Source: CAD feature listing. Evaluate the final solid. Frame: model axes, mm. A direction names the side the tool comes from. Give positions to 0.01 mm unless a question says otherwise; leave off trailing zeros. Write each loop counter-clockwise with the first axis right and the second up, starting at its lowest first coordinate (ties: lowest second). Pieces come first, ordered by that corner, then holes. Notation, with made-up numbers: (88, -40) -> (101, -40) arc R8 ccw to (101, -26) -> close; hole circle Ø1 at (-10, -7.5). An arc over 180 degrees is marked (long way). Write item = value, one per line.
Autodesk Inventor part; units mm, degrees
ref_plane "YZ Plane" through (0, 0, 0) normal (1, 0, 0) x (0, 1, 0)
ref_plane "XY Plane" through (0, 0, 0) normal (0, 0, 1) x (1, 0, 0)
ref_plane "UCS1: YZ Plane" through (0, 0, 0) normal (1, 0, 0) x (0, 1, 0)
sketch "Sketch2" plane through (0, 0, 0) normal (1, 0, 0) x (0, 1, 0)
  circle A0 centre (0, -70) radius 26
  line L0 (25, -200) -> (-25, -200)
  line L1 (0, -70) -> (0, -200) construction
  line L2 (-25.9992, -70.2001) -> (-25, -200)
  line L3 (25.9992, -70.2001) -> (25, -200)
  circle A1 centre (0, 0) radius 17.5
  circle A2 centre (0, -70) radius 17.5
  line L4 (17.5, 0) -> (17.5, -70)
  line L5 (-17.5, 0) -> (-17.5, -70)
  dimension "d1" = 52
  dimension "d3" = 50
  dimension "d25" = 130
  dimension "d26" = 35
  dimension "d27" = 70
extrude "Extrusion1" add sketch "Sketch2" against normal blind 45 contours A0 L5 A2 L4 | A0 L4 A2 L5 | A2
extrude "Extrusion2" add sketch "Sketch2" along normal blind 45 from surface at -45 contours A0 L3 L0 L2
sketch "Sketch5" plane through (-45, -25, -200) normal (0, 0, -1) x (-1, 0, 0)
  circle A0 centre (-22.5, 25) radius 10
  line L0 (-45, 50) -> (-45, 0)
  line L1 (-45, 50) -> (0, 50)
  point P0 (-45, 25)
  point P1 (-45, 25)
  point P2 (45, 0)
  point P3 (-22.5, 50)
  dimension "d22" = 20
extrude "Extrusion4" cut sketch "Sketch5" against normal blind 60
ref_plane "Work Plane1" through (-22.5, 0, -70) normal (1, 0, 0) x (0, 0, -1)
sketch "Sketch4" plane through (-22.5, 0, -70) normal (1, 0, 0) x (0, 0, -1)
  line L0 (130, 25) -> (130, -25)
  arc A0 (125.9592, -40) -> (130, 0) centre (-70, 0) ccw
  line L1 (125.9592, -40) -> (130, -40)
  line L2 (130, -40) -> (130, 0)
  line L3 (201.2, 0) -> (-115.2, 0)
  line L4 (-70, 0) -> (130, 0)
  point P0 (-70, 0)
  point P1 (156, -25)
  point P2 (156, 25)
  point P3 (156, -25)
  point P4 (-25, -130)
  point P5 (25, -130)
  dimension "d18" = 40
revolve "Revolution1" cut sketch "Sketch4" angle 360 about axis through (-22.5, 0, 0) along (0, 0, -1)
extrude "Extrusion5" add sketch "Sketch2" along normal blind 12 contours L5 A1 L4 A0 | A0 L4 A2 L5 | A1 | A2 picked at (-13.2429, -51.1519)
properties part number "shank_inventor"
(1) Access query for faces 5 (the face through (6, 17.5, -35)), 6 (the face through (5.916, 0.385, -87.496)), 7 (the face through (12, 0, -34)), 8 (the face through (6, -17.5, -35)). Directions: +Z, -Z, +X, -X, +Y, -Y. A direction counts if a zero-diameter tool reaches every point of the face in a straight line with its end or side. Return the directions, or none.
Values follow:
face_5 = +Z, -Z, +X, +Y
face_6 = -Z, +X
face_7 = +Z, -Z, +X, +Y, -Y
face_8 = +Z, -Z, +X, -Y
(2) Section query A-A (z = -32). Return loops of the section in (x, y).
Values follow:
outline = (0, -17.5) -> (12, -17.5) -> (12, 17.5) -> (0, 17.5) -> close
(3) Pull-direction query (Y, two-part tool) for faces 1 (the face through (5.916, -0.385, 17.496)), 2 (the face through (-22, 0, -140)), 3 (the face through (-32.04, 3, -170.29)), 4 (the face through (0, 0, -16)); classes: pulls with the +Y half, pulls with the -Y half, needs draft (parallel to the pull), parting line crosses it, or undercut.
Values follow:
face_1 = parting line crosses it
face_2 = undercut
face_3 = undercut
face_4 = needs draft
(4) Material intervals for line 1 (X direction, y = 0, z = -156); line 2 (X direction, y = 23.5, z = -184.5); line 3 (X direction, y = -12, z = -17.5), sorted ascending.
Values follow:
line_1 = -45 to -32.5, -12.5 to 0
line_2 = -45 to 0
line_3 = 0 to 12
(5) First-contact query: pin 1 (6 mm diameter, centred on x = -26, z = -169, fed in from +Y); pin 2 (9.5 mm diameter, centred on x = 4.5, z = -35.5, fed in from +Y); pin 3 (1.5 mm diameter, centred on x = -18, y = -15, fed in from +Z). Flat tips, straight axial feed; report the tip coordinate or a pass-through.
Values follow:
pin_1 = 25.26
pin_2 = 17.5
pin_3 = -48.25
